from build123d import *

# Parameters (mm, degrees)
F0_R     = 7.5
F1_DEPTH = 3
F2_R     = 7.5
F3_DEPTH = 5
F0_R_2   = 1.5
F4_DEPTH = 25


with BuildPart() as f1:
    # F0 (on Top) → F1 (new body)
    with BuildSketch(Plane.XY):
        with Locations((7.5, 7.5)):
            Circle(F0_R)
        Polygon((7.5, 10.9641016151), (10.5, 9.2320508076), (10.5, 5.7679491924), (7.5, 4.0358983849), (4.5, 5.7679491924), (4.5, 9.2320508076), align=None, mode=Mode.SUBTRACT)
    extrude(amount=F1_DEPTH)

    # F2 (on face) → F3 (join)
    with BuildSketch(Plane.XY.offset(3)):
        with Locations((7.5, 7.5)):
            Circle(F2_R)
        Polygon((4.5, 5.7679491924), (4.5, 9.2320508076), (7.5, 10.9641016151), (10.5, 9.2320508076), (10.5, 5.7679491924), (7.5, 4.0358983849), align=None, mode=Mode.SUBTRACT)
        Polygon((7.5, 10.9641016151), (4.5, 9.2320508076), (4.5, 5.7679491924), (7.5, 4.0358983849), (10.5, 5.7679491924), (10.5, 9.2320508076), align=None)
    extrude(amount=F3_DEPTH)

    # F0 (on Top) → F4 (cut)
    with BuildSketch(Plane.XY):
        with Locations((7.5, 7.5)):
            Circle(F0_R_2)
    extrude(amount=F4_DEPTH, mode=Mode.SUBTRACT)


solid = f1.part
Geometry: final body of the model. Coordinates: model frame, mm. A direction names the side the tool comes from. Coordinates: 2 decimals unless noted, no trailing zeros. Loops run counter-clockwise (first coordinate to the right, second up) from the corner with the lowest first, then second, coordinate; pieces in that order, holes last. Notation, with made-up numbers: (37, -38) - (73, -38) arc R21 cw to (73, -23) - close; hole circle Ø2 at (33.25, 14.25). An arc over 180 degrees is marked (long way). Put each result on its own line as item: value. Start each with the question number.
Q1. Cut plane D-D, the plane y = 10. Return loops of the section in (x, z), and give its area (3 significant figures).
Q2. Pin query (flat end, axial travel): pin 1 Ø3 at (x, z) = (13.5, 2.5) entering from -Y; pin 2 Ø1.5 at (y, z) = (6.5, 2) entering from +X; pin 3 Ø3 at (x, y) = (7.5, 8) entering from -Z. Return the tip coordinate at first contact, or that it passes through.
Q3. Pull-direction query (X, two-part tool) for faces 1 (the flat face through (6.8, 6, 3)), 2 (the flat face through (7.4, 9.3, 8)), 3 (the cylindrical face through (1.548, 2.936, 3.944)), 4 (the flat face through (6, 4.9, 1.5)); classes: released by +X, released by -X, zero draft, split by the parting line, or undercut.
Q4. Cut plane C-C, the plane z = 0.75. Return loops of the section in (x, y).
Q5. Line query: line 1 (Y direction, x = 7.5, z = 5.3); line 2 (X direction, y = 4.25, z = 1.75); line 3 (Y direction, x = 7, z = 3.5). Output: solid intervals per line, ascending.
Q6. Set-up query: faces 5 (the cylindrical face through (6.3, 6.6, 5.5)), 6 (the flat face through (9, 4.9, 1.5)). Return all of +Z, -Z, +X, -X, +Y, -Y with unobstructed straight access to the full face (end or side cutting, diameter ignored); none if empty.
Q7. Cut plane B-B, the plane x = 7. Return loops of the section in (y, z), and give its area (3 significant figures).
Q8. Cut plane A-A, the plane y = 7.5. Return loops of the section in (x, z), and give its area (3 significant figures).
Filled sheet:
1. outline: (0.43, 0) - (5.83, 0) - (5.83, 3) - (9.17, 3) - (9.17, 0) - (14.57, 0) - (14.57, 8) - (0.43, 8) - close
1. area: 103 mm²
2. pin 1: y = 1.5
2. pin 2: x = 15
2. pin 3: z = 3
3. face 1: undercut
3. face 2: zero draft
3. face 3: split by the parting line
3. face 4: undercut
4. outline: circle Ø15 at (7.5, 7.5); hole (4.5, 5.77) - (7.5, 4.04) - (10.5, 5.77) - (10.5, 9.23) - (7.5, 10.96) - (4.5, 9.23) - close
5. line 1: 0 to 6, 9 to 15
5. line 2: 0.74 to 7.13, 7.87 to 14.26
5. line 3: 0.02 to 6.09, 8.91 to 14.98
6. face 5: +Z, -Z
6. face 6: -Z
7. outline: (0.02, 0) - (4.32, 0) - (4.32, 3) - (6.09, 3) - (6.09, 8) - (0.02, 8) - close; (8.91, 3) - (10.68, 3) - (10.68, 0) - (14.98, 0) - (14.98, 8) - (8.91, 8) - close
7. area: 86.5 mm²
8. outline: (0, 0) - (4.5, 0) - (4.5, 3) - (6, 3) - (6, 8) - (0, 8) - close; (9, 3) - (10.5, 3) - (10.5, 0) - (15, 0) - (15, 8) - (9, 8) - close
8. area: 87.0 mm²
